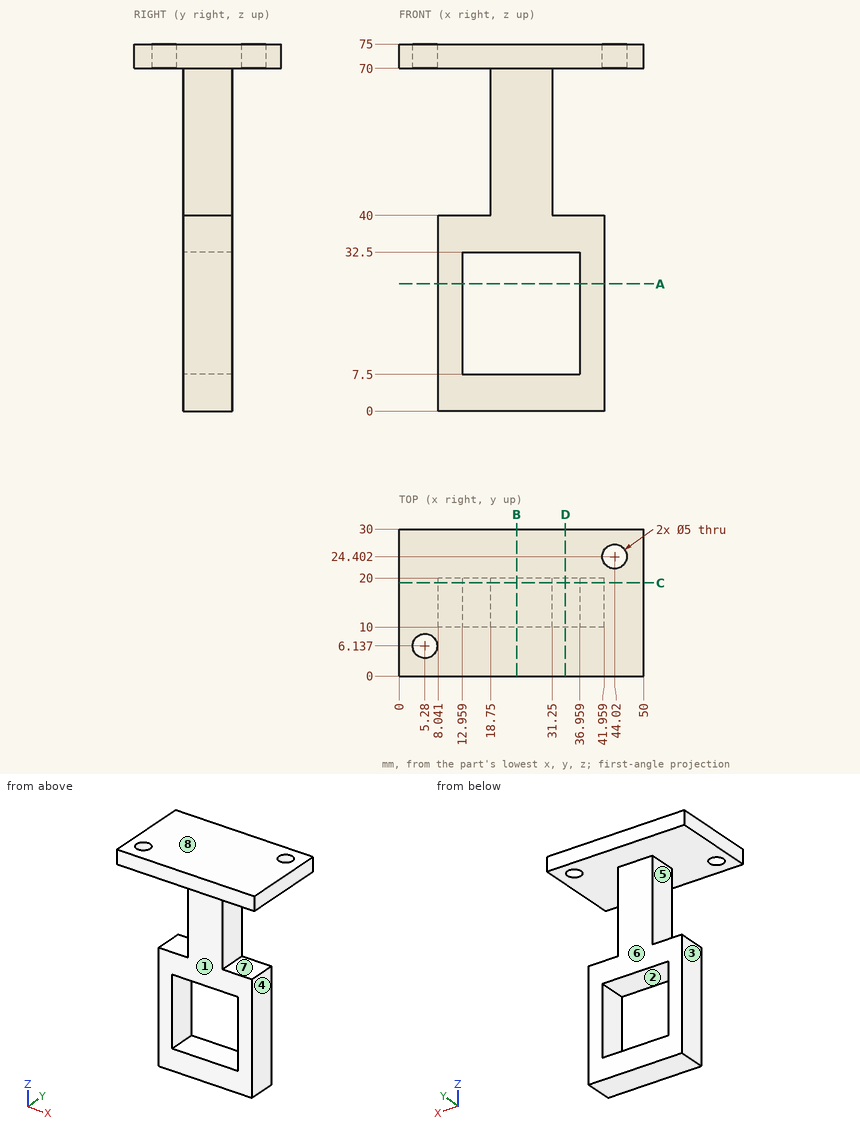
Geometry: see drawing. Coordinates: mm, zero at the bounding-box minimum. A direction names the side the tool comes from. Give positions to 0.01 mm unless a question says otherwise; leave off trailing zeros. Order: outer loops, then holes, each group sorted by start corner. A loop starts at its lowest first (then second) coordinate and runs counter-clockwise, first axis right, second up. Notation, with made-up numbers: (77.25, 65) - (135.25, 65) arc R32 ccw to (135.25, 101) - close; hole circle Ø9 at (59, 58.25). An arc over 180 degrees is marked (long way). Write each question's results on one line, items separated by ' | '.
Item 1: Access query for the marked faces 1, 2, 3, 4 and 5. Directions: +Z, -Z, +X, -X, +Y, -Y. A direction counts if a zero-diameter tool reaches every point of the face in a straight line with its end or side. Return the directions, or none.
A:
face 1: -Z, +X, -X, -Y | face 2: +Y, -Y | face 3: -Z, -X, +Y, -Y | face 4: -Z, +X, +Y, -Y | face 5: -X, +Y, -Y
Item 2: Section A-A (z = 26). Return loops of the section in (x, y).
A:
outline: (8.04, 10) - (12.96, 10) - (12.96, 20) - (8.04, 20) - close; (36.96, 10) - (41.96, 10) - (41.96, 20) - (36.96, 20) - close
Item 3: Draft query along Z for the marked faces 6, 7 and 8. Return one class per face: released by +Z, released by -Z, zero draft, split by the parting line, or undercut.
A:
face 6: zero draft | face 7: undercut | face 8: released by +Z
Item 4: Section B-B (x = 24). Return loops of the section in (y, z), and give its area (3 significant figures).
A:
outline: (0, 70) - (10, 70) - (10, 32.5) - (20, 32.5) - (20, 70) - (30, 70) - (30, 75) - (0, 75) - close; (10, 0) - (20, 0) - (20, 7.5) - (10, 7.5) - close | area: 600 mm^2
Item 5: Contact query for flat-ended pins moving along their axis: pin 1 Ø6 at (x, z) = (38, 27.5) entering from +Y; pin 2 Ø6.5 at (x, y) = (5.28, 6.14) entering from +Z; pin 3 Ø11 at (y, z) = (15, 21.5) entering from +X; pin 4 Ø8 at (y, z) = (13, 19) entering from -X. Output: stop coordinate, or through.
A:
pin 1: stops at y = 20 | pin 2: stops at z = 75 | pin 3: stops at x = 41.96 | pin 4: stops at x = 8.04
Item 6: Material intervals for line 1 along Z through (x, y) = (34, 17.75); line 2 along Z through (x, y) = (41, 18.5); line 3 along Z through (x, y) = (26.5, 13), sorted ascending.
A:
line 1: z = 0 to 7.5, 32.5 to 40, 70 to 75 | line 2: z = 0 to 40, 70 to 75 | line 3: z = 0 to 7.5, 32.5 to 75
Item 7: Section C-C (y = 19). Return loops of the section in (x, z), and give its area (3 significant figures).
A:
outline: (0, 70) - (18.75, 70) - (18.75, 40) - (8.04, 40) - (8.04, 0) - (41.96, 0) - (41.96, 40) - (31.25, 40) - (31.25, 70) - (50, 70) - (50, 75) - (0, 75) - close; hole (12.96, 7.5) - (36.96, 7.5) - (36.96, 32.5) - (12.96, 32.5) - close | area: 1,380 mm^2
Item 8: Section D-D (x = 34). Return loops of the section in (y, z), and give its area (3 significant figures).
A:
outline: (0, 70) - (30, 70) - (30, 75) - (0, 75) - close; (10, 0) - (20, 0) - (20, 7.5) - (10, 7.5) - close; (10, 32.5) - (20, 32.5) - (20, 40) - (10, 40) - close | area: 300 mm^2
